Design review of the part built by this model. Coordinates are the model's own, in mm. A direction names the side the tool comes from. Coordinates: 2 decimals unless noted, no trailing zeros. Write each loop counter-clockwise with the first axis right and the second up, starting at its lowest first coordinate (ties: lowest second). Pieces come first, ordered by that corner, then holes.
Q1. Take a section at C-C (x = 13.25). Give the boundary of the cut face in (y, z), and give its area (3 significant figures).
Q2. Take a section at A-A (x = 17). Give the boundary of the cut face in (y, z), and give its area (4 significant figures).
Q3. Machinability: for faces 5 (the flat face through (10, 5, 0)), 6 (the flat face through (10, -5, 0)), 7 (the flat face through (4.136, 1.355, 8.766)), which of the approach directions +Z, -Z, +X, -X, +Y, -Y give a long, thin tool a straight path to every point of the face, cutting with its end or side? Answer none if there is none.
Q4. Take a section at B-B (x = 4). Give the boundary of the cut face in (y, z), and give its area (3 significant figures).
Q5. Take a section at D-D (y = 0.5). Give the boundary of the cut face in (x, z).
Q6. Insertion check: pin 1 (5 mm diameter, centred on x = 17, y = -3.173, fed in from -Z); pin 2 (2.5 mm diameter, centred on x = 3, y = -6.673, fed in from -Z); pin 3 (1 mm diameter, centred on x = 12, y = 5.5, fed in from +Z). Each pin has a flat end and moves straight along its axis. Give the tip position at first contact, or say it passes through.
Q7. For probe 1 along Y at (x, z) = (3, -1.45); probe 2 along Z at (x, y) = (5.75, 8.5); probe 3 along Y at (x, z) = (6.75, 2), list the stretches that pass through material, from the lowest coordinate up.
Q8. Mouldability with a two-part tool opening along Y and no side actions: class faces 1 (the flat face through (9.86, 7.535, -0.986)), 2 (the flat face through (7.3, -1.75, 7.97)), 3 (the cylindrical face through (18.5, -3.1, -1)), 4 (the flat face through (0, 3, 8)) as pulls with the +Y half, pulls with the -Y half, needs draft (parallel to the pull), parting line crosses it, or undercut.
Autodesk Inventor part; units mm, degrees
ref_plane "YZ Plane" through (0, 0, 0) normal (1, 0, 0) x (0, 1, 0)
ref_plane "XZ Plane" through (0, 0, 0) normal (0, 1, 0) x (-1, 0, 0)
ref_plane "XY Plane" through (0, 0, 0) normal (0, 0, 1) x (1, 0, 0)
sketch "草图1" plane through (0, 0, 0) normal (0, 0, 1) x (1, 0, 0)
  line L0 (0, 5) -> (20, 0)
  line L1 (20, 0) -> (0, -5)
  line L2 (0, -5) -> (0, 5)
  point P0 (0, 0)
  point P1 (0, 0)
  dimension "d0" = 10
  dimension "d1" = 20
sketch "草图2" plane through (0, 0, 0) normal (1, 0, 0) x (0, 1, 0)
  point P0 (0, 0)
  point P1 (0, 28)
  dimension "d2" = 28
loft "放样1" add profiles "草图1" section 2 point at (0, 0, 28)
shell "抽壳1" thickness 1 removed faces 2 at (6.6667, 0, 0) at (0, 0, 9.3333)
sketch "草图3" plane through (0, 3.9539, 0) normal (0, 0, -1) x (-1, 0, 0)
  line L0 (0, -13.9539) -> (-20, -13.9539)
  line L1 (-20, -13.9539) -> (-20, 6.0461)
  line L2 (-20, 6.0461) -> (0, 6.0461)
  line L3 (0, 6.0461) -> (0, -13.9539)
  line L4 (0, -13.9539) -> (-20, -8.9539)
  line L5 (0, 6.0461) -> (-20, 1.0461)
  line L6 (-20, -3.9539) -> (0, -8.9539)
  line L7 (0, 1.0461) -> (-20, -3.9539)
  point P0 (0, -3.9539)
  point P1 (0, -3.9539)
  dimension "d8" = 20
extrude "拉伸1" add sketch "草图3" along normal blind 2 contours L4 L1 L6 L3 | L6 L7 L3 | L7 L1 L5 L3
sketch "草图4" plane through (0, 3.9539, -2) normal (0, 0, -1) x (-1, 0, 0)
  circle A0 centre (-3, -10.6269) radius 1.5
  line L0 (-20, -8.9539) -> (0, -13.9539)
  circle A1 centre (-17, -7.1269) radius 1.5
  circle A2 centre (-3, 2.7192) radius 1.5
  circle A3 centre (-17, -0.7808) radius 1.5
  line L1 (0, 6.0461) -> (-20, 1.0461)
  line L2 (-20, 1.0461) -> (-20, -8.9539)
  line L3 (0, -13.9539) -> (0, 6.0461)
  point P0 (0, -3.9539)
  dimension "d11" = 3
  dimension "d12" = 2.5
  dimension "d13" = 3
  dimension "d14" = 3
  dimension "d15" = 3
  dimension "d16" = 2.5
  dimension "d17" = 2.5
  dimension "d18" = 2.5
  dimension "d19" = 3
  dimension "d20" = 3
  dimension "d21" = 3
  dimension "d22" = 3
extrude "拉伸2" cut sketch "草图4" against normal through all contours A0 | A1 | A2 | A3
properties part number "分离前导形片"
Response:
1. outline: (-6.69, -2) - (6.69, -2) - (6.69, 0) - (1.69, 0) - (0, 9.45) - (-1.69, 0) - (-6.69, 0) - close; hole (-0.64, 0) - (0.64, 0) - (0, 3.59) - close
1. area: 40.4 mm2
2. outline: (-5.75, -2) - (-4.67, -2) - (-4.67, 0) - (-5.75, 0) - close; (-1.67, -2) - (1.67, -2) - (1.67, 0) - (0.75, 0) - (0, 4.2) - (-0.75, 0) - (-1.67, 0) - close; (4.67, -2) - (5.75, -2) - (5.75, 0) - (4.67, 0) - close
2. area: 14.15 mm2
3. face 5: +Z, +X, +Y
3. face 6: +Z, +X, -Y
3. face 7: -X
4. outline: (-9, -2) - (-7.79, -2) - (-7.79, 0) - (-9, 0) - close; (-5.55, -2) - (5.56, -2) - (5.56, 0) - (4, 0) - (0, 22.4) - (-4, 0) - (-5.55, 0) - close; (7.79, -2) - (9, -2) - (9, 0) - (7.79, 0) - close; hole (-2.95, 0) - (2.95, 0) - (0, 16.54) - close
4. area: 67.8 mm2
5. outline: (0, -2) - (20, -2) - (20, 0) - (18, 0) - (0, 25.2) - (0, 19.34) - (13.82, 0) - (0, 0) - close
6. pin 1: stops at z = -2
6. pin 2: passes through
6. pin 3: stops at z = 0
7. probe 1: y = -9.25 to -8.17, -5.17 to 5.17, 8.17 to 9.25
7. probe 2: z = -2 to 0
7. probe 3: y = -2.96 to -1.91, 1.91 to 2.96
8. face 1: pulls with the +Y half
8. face 2: pulls with the -Y half
8. face 3: undercut
8. face 4: needs draft
